Autodesk Inventor part; units mm, degrees
ref_plane "YZ Plane" through (0, 0, 0) normal (1, 0, 0) x (0, 1, 0)
ref_plane "XZ Plane" through (0, 0, 0) normal (0, 1, 0) x (-1, 0, 0)
ref_plane "XY Plane" through (0, 0, 0) normal (0, 0, 1) x (1, 0, 0)
sketch "Sketch1" plane through (0, 0, 0) normal (0, 1, 0) x (-1, 0, 0)
  arc A0 (-147.5, 0) -> (147.5, 0) centre (0, 0) ccw
  line L0 (-147.5, 0) -> (-147.5, 122.1)
  line L1 (-122.1, 147.5) -> (122.1, 147.5)
  line L2 (147.5, 122.1) -> (147.5, 0)
  arc A1 (-122.1, 147.5) -> (-147.5, 122.1) centre (-122.1, 122.1) ccw
  arc A2 (147.5, 122.1) -> (122.1, 147.5) centre (122.1, 122.1) ccw
  point P0 (-147.5, 147.5)
  point P1 (147.5, 147.5)
  dimension "d0" = 295
  dimension "d98" = 147.5
  dimension "d99" = 147.5
  dimension "d101" = 295
  dimension "d102" = 147.5
  dimension "d217" = 25.4
extrude "Extrusion1" add sketch "Sketch1" along normal blind 5
sketch "Sketch8" plane through (0, 5, 0) normal (0, 1, 0) x (1, 0, 0)
  circle A0 centre (76.2, -76.2) radius 1.7
  circle A1 centre (76.2, 76.2) radius 1.7
  circle A2 centre (-76.2, 76.2) radius 1.7
  circle A3 centre (-76.2, -76.2) radius 1.7
  arc A4 (147.5, 0) -> (-147.5, 0) centre (0, 0) ccw construction
  line L0 (0, 147.5) -> (0, -147.5) construction
  line L1 (-122.1, -147.5) -> (122.1, -147.5) construction
  line L2 (-147.5, 0) -> (-147.5, -122.1) construction
  line L3 (147.5, -122.1) -> (147.5, 0) construction
  line L4 (-147.5, 0) -> (147.5, 0) construction
  point P0 (0, 0)
  point P1 (-177, -177)
  point P2 (177, -177)
  point P3 (122.1, -147.5)
  dimension "d103" = 3.4
  dimension "d104" = 3.4
  dimension "d105" = 3.4
  dimension "d106" = 3.4
  dimension "d115" = 76.2
  dimension "d116" = 76.2
  dimension "d117" = 76.2
  dimension "d118" = 76.2
  dimension "d119" = 76.2
  dimension "d120" = 76.2
  dimension "d121" = 76.2
  dimension "d122" = 76.2
extrude "Stand-Offs" cut sketch "Sketch8" against normal through all
sketch "Sketch9" plane through (0, 5, 0) normal (0, 1, 0) x (1, 0, 0)
  line L0 (-131.6, -54.8) -> (-131.6, -134.8)
  line L1 (-131.6, -134.8) -> (-101.6, -134.8)
  line L2 (-101.6, -134.8) -> (-101.6, -54.8)
  line L3 (-101.6, -54.8) -> (-131.6, -54.8)
  circle A0 centre (-95.25, -69.4) radius 1.7
  circle A1 centre (-95.25, -120.2) radius 1.7
  circle A2 centre (-137.95, -120.2) radius 1.7
  circle A3 centre (-137.95, -69.4) radius 1.7
  arc A4 (147.5, 0) -> (-147.5, 0) centre (0, 0) ccw construction
  line L4 (0, 147.5) -> (0, -147.5) construction
  line L5 (-122.1, -147.5) -> (122.1, -147.5) construction
  line L6 (-177, -177) -> (177, -177) construction
  line L7 (-101.6, -94.8) -> (-131.6, -94.8) construction
  line L8 (131.6, -134.8) -> (101.6, -134.8)
  line L9 (101.6, -134.8) -> (101.6, -54.8)
  line L10 (101.6, -54.8) -> (131.6, -54.8)
  circle A5 centre (95.25, -69.4) radius 1.7
  circle A6 centre (95.25, -120.2) radius 1.7
  line L11 (131.6, -54.8) -> (131.6, -134.8)
  circle A7 centre (137.95, -69.4) radius 1.7
  circle A8 centre (137.95, -120.2) radius 1.7
  line L12 (101.6, -94.8) -> (131.6, -94.8) construction
  point P0 (177.1241, 0)
  point P1 (122.1, -147.5)
  dimension "d126" = 30
  dimension "d129" = 3.4
  dimension "d130" = 3.4
  dimension "d131" = 3.4
  dimension "d132" = 3.4
  dimension "d133" = 6.35
  dimension "d134" = 6.35
  dimension "d135" = 6.35
  dimension "d136" = 6.35
  dimension "d141" = 101.6
  dimension "d142" = 12.7
  dimension "d143" = 80
  dimension "d144" = 25.4
  dimension "d145" = 25.4
  dimension "d146" = 25.4
  dimension "d147" = 25.4
extrude "Wheels" cut sketch "Sketch9" against normal through all
sketch "Sketch10" plane through (0, 5, 0) normal (0, 1, 0) x (1, 0, 0)
  circle A0 centre (-51.06, -108.2493) radius 1.7
  circle A1 centre (-9.2516, -108.2493) radius 1.7
  circle A2 centre (-51.06, -81.3507) radius 1.7
  circle A3 centre (-9.2516, -81.3507) radius 1.7
  arc A4 (147.5, 0) -> (-147.5, 0) centre (0, 0) ccw construction
  line L0 (0, 147.5) -> (0, -147.5) construction
  line L1 (-122.1, -147.5) -> (122.1, -147.5) construction
  line L2 (147.5, -122.1) -> (147.5, 0) construction
  line L3 (-147.5, 0) -> (-147.5, -122.1) construction
  line L4 (147.5, 0) -> (-147.5, 0) construction
  line L5 (-131.6, -54.8) -> (-131.6, -134.8) construction
  line L6 (-131.6, -94.8) -> (131.6, -94.8) construction
  line L7 (131.6, -54.8) -> (131.6, -134.8) construction
  line L8 (-101.6, -54.8) -> (-101.6, -134.8) construction
  circle A5 centre (51.06, -108.2493) radius 1.7
  circle A6 centre (51.06, -81.3507) radius 1.7
  circle A7 centre (9.2516, -108.2493) radius 1.7
  circle A8 centre (9.2516, -81.3507) radius 1.7
  point P0 (-177, -177)
  point P1 (177, -177)
  point P2 (122.1, -147.5)
  dimension "d150" = 3.4
  dimension "d151" = 3.4
  dimension "d152" = 3.4
  dimension "d153" = 3.4
  dimension "d154" = 26.8986
  dimension "d155" = 26.8986
  dimension "d156" = 41.8084
  dimension "d157" = 41.8084
  dimension "d161" = 50.54
  dimension "d162" = 13.4493
  dimension "d163" = 13.4493
  dimension "d166" = 13.4493
  dimension "d167" = 13.4493
extrude "Motor Mount" cut sketch "Sketch10" against normal through all
sketch "Sketch11" plane through (0, 5, 0) normal (0, 1, 0) x (1, 0, 0)
  circle A0 centre (-46.25, 39.25) radius 1.7
  circle A1 centre (46.25, 39.25) radius 1.7
  circle A2 centre (46.25, -39.25) radius 1.7
  circle A3 centre (-46.25, -39.25) radius 1.7
  line L0 (-147.5, 0) -> (-147.5, -122.1) construction
  arc A4 (147.5, 0) -> (-147.5, 0) centre (0, 0) ccw construction
  line L1 (-147.5, 0) -> (147.5, 0) construction
  line L2 (0, 147.5) -> (0, -147.5) construction
  line L3 (-122.1, -147.5) -> (122.1, -147.5) construction
  point P0 (-177, -177)
  point P1 (177, -177)
  point P2 (122.1, -147.5)
  dimension "d170" = 3.4
  dimension "d171" = 3.4
  dimension "d172" = 3.4
  dimension "d173" = 3.4
  dimension "d174" = 92.5
  dimension "d175" = 92.5
  dimension "d176" = 78.5
  dimension "d177" = 78.5
  dimension "d183" = 46.25
  dimension "d184" = 39.25
  dimension "d185" = 39.25
  dimension "d186" = 46.25
  dimension "d235" = 46.25
extrude "PCB" cut sketch "Sketch11" against normal through all
sketch "Sketch12" plane through (0, 5, 0) normal (0, 1, 0) x (1, 0, 0)
  circle A0 centre (20, 103.05) radius 1.7
  circle A1 centre (-20, 103.05) radius 1.7
  line L0 (-147.5, 0) -> (-147.5, -122.1) construction
  arc A2 (147.5, 0) -> (-147.5, 0) centre (0, 0) ccw construction
  line L1 (-147.5, 0) -> (147.5, 0) construction
  arc A3 (147.5, 0) -> (-147.5, 0) centre (0, 0) ccw construction
  line L2 (0, 147.5) -> (0, -147.5) construction
  point P0 (-177, -177)
  point P1 (0, 147.5)
  dimension "d190" = 3.4
  dimension "d191" = 3.4
  dimension "d192" = 40
  dimension "d198" = 44.45
  dimension "d200" = 44.45
  dimension "d201" = 20
extrude "Ball Caster" cut sketch "Sketch12" against normal through all
sketch "Sketch13" plane through (0, 5, 0) normal (0, 1, 0) x (1, 0, 0)
  line L0 (-34.925, 119.3) -> (-28.575, 119.3)
  line L1 (-28.575, 119.3) -> (-28.575, 114.3)
  line L2 (-28.575, 114.3) -> (-34.925, 114.3)
  line L3 (-34.925, 114.3) -> (-34.925, 119.3)
  line L4 (-22.225, 119.3) -> (-15.875, 119.3)
  line L5 (-15.875, 119.3) -> (-15.875, 114.3)
  line L6 (-15.875, 114.3) -> (-22.225, 114.3)
  line L7 (-22.225, 114.3) -> (-22.225, 119.3)
  line L8 (-9.525, 119.3) -> (-3.175, 119.3)
  line L9 (-3.175, 119.3) -> (-3.175, 114.3)
  line L10 (-3.175, 114.3) -> (-9.525, 114.3)
  line L11 (-9.525, 114.3) -> (-9.525, 119.3)
  line L12 (3.175, 119.3) -> (9.525, 119.3)
  line L13 (9.525, 119.3) -> (9.525, 114.3)
  line L14 (9.525, 114.3) -> (3.175, 114.3)
  line L15 (3.175, 114.3) -> (3.175, 119.3)
  line L16 (15.875, 119.3) -> (22.225, 119.3)
  line L17 (22.225, 119.3) -> (22.225, 114.3)
  line L18 (22.225, 114.3) -> (15.875, 114.3)
  line L19 (15.875, 114.3) -> (15.875, 119.3)
  line L20 (28.575, 119.3) -> (34.925, 119.3)
  line L21 (34.925, 119.3) -> (34.925, 114.3)
  line L22 (34.925, 114.3) -> (28.575, 114.3)
  line L23 (28.575, 114.3) -> (28.575, 119.3)
  arc A0 (147.5, 0) -> (-147.5, 0) centre (0, 0) ccw construction
  line L24 (0, 147.5) -> (0, -147.5) construction
  line L25 (-122.1, -147.5) -> (122.1, -147.5) construction
  line L26 (147.5, -122.1) -> (147.5, 0) construction
  line L27 (-147.5, 0) -> (-147.5, -122.1) construction
  line L28 (147.5, 0) -> (-147.5, 0) construction
  point P0 (-177, -177)
  point P1 (177, -177)
  point P2 (122.1, -147.5)
  dimension "d204" = 5
  dimension "d205" = 6.35
  dimension "d208" = 12.7
  dimension "d213" = 114.3
  dimension "d214" = 3.175
extrude "Switch" cut sketch "Sketch13" against normal through all
equation "\"d101\" = d0"
equation "\"m3_heat_set_insert\" = 4"
equation "\"m3_clearance\" = 3.4"
equation "\"m3_heat_set_depth\" = 7"
equation "\"hardboard_thickness\" = 5"
equation "\"robot_diameter\" = 354"
properties part number "layer1_new_300mm"
For this review, take the finished solid that the model builds, in its own axes (mm). Round coordinates to 2 decimals unless told otherwise and drop trailing zeros. Order: outer loops, then holes, each group sorted by start corner. A loop starts at its lowest first (then second) coordinate and runs counter-clockwise, first axis right, second up. Notation, with made-up numbers: (19.5, 60) -> (71.5, 60) arc R30 cw to (71.5, 95) -> close; hole circle Ø5 at (20, 31.25). An arc over 180 degrees is marked (long way). Write item = value, one per line. Start each with the question number.
1) Insertion check: pin 1 (2.5 mm diameter, centred on y = 3.5, z = -116, fed in from +X); pin 2 (3 mm diameter, centred on x = -91, z = -75, fed in from -Y); pin 3 (1.5 mm diameter, centred on x = -17.5, y = 1.5, fed in from -Z); pin 4 (2.5 mm diameter, centred on y = 1.5, z = -115.5, fed in from +X). Each pin has a flat end and moves straight along its axis. Give the tip position at first contact, or say it passes through.
2) Take a section at A-A on x = -126. State the section outline as (y, z) points, plus the area to 3 significant figures.
3) Take a section at C-C on z = -88. State the section outline as (x, y) points.
4) Take a section at B-B on y = 4.05. Count the separate pieces of the cut face and the enclosed holes in it, plus the area to 3 significant figures.
5) To check wall thickness, follow line 1 (X direction, y = 0.6, z = 88); line 2 (X direction, y = 2.5, z = 132); line 3 (Z direction, x = 126.5, y = 2.75). State the ranges of each line that lie inside material, in increasing order. Write a range as from..to.
Verdict:
q1.pin_1 = 92.68
q1.pin_2 = 0
q1.pin_3 = -146.55
q1.pin_4 = 93.29
q2.outline = (0, -76.68) -> (5, -76.68) -> (5, 54.8) -> (0, 54.8) -> close; (0, 134.8) -> (5, 134.8) -> (5, 147.2) -> (0, 147.2) -> close
q2.area = 719 mm2
q3.outline = (-118.37, 0) -> (118.37, 0) -> (118.37, 5) -> (-118.37, 5) -> close
q4.separate_pieces = 1
q4.enclosed_holes = 34
q4.area = 72,200 mm2
q5.line_1 = -147.5..-131.6, -101.6..101.6, 131.6..147.5
q5.line_2 = -145.49..-131.6, -101.6..101.6, 131.6..145.49
q5.line_3 = -75.86..54.8, 134.8..147.12
